Here's how the part is built. I have some questions about the finished solid (model axes, mm). A direction names the side the tool comes from. Coordinates: 2 decimals unless noted, no trailing zeros. Loops run counter-clockwise (first coordinate to the right, second up) from the corner with the lowest first, then second, coordinate; pieces in that order, holes last. Notation, with made-up numbers: (52, 67.5) -> (88, 67.5) arc R12 cw to (88, 88.5) -> close; hole circle Ø3 at (5, 21). An arc over 180 degrees is marked (long way). Answer as a JSON object with one key per item and string values. Group by question number.
Q1. I want a section at D-D on x = -6.5. Write out the boundary of the cut face in (y, z) (1 decimal), then the cut area to 3 significant figures.
Q2. On a 3-axis mill with a long thin cutter (end or side, diameter ignored), from which of +Z, -Z, +X, -X, +Y, -Y can I reach the whole of each face in a straight line? I mean faces 1 (the cylindrical face through (-2.75, 12.4, 21.57)), 2 (the cylindrical face through (-7.559, -5.796, 23.982)), 3 (the cylindrical face through (-0.69, 3.1, 9.08)). Say none if no direction works.
Q3. I'm going to push flat-ended pins straight in: pin 1 (5 mm diameter, centred on x = 3, z = 15.5, fed in from +Y); pin 2 (5 mm diameter, centred on y = -1.5, z = 6.5, fed in from -X) (3 decimals); pin 3 (8 mm diameter, centred on y = 7.5, z = 20, fed in from -X). Where does each tip first touch, or does it pass through?
Q4. I want a section at A-A on x = 0. Write out the boundary of the cut face in (y, z) (1 decimal).
Q5. I need wall thicknesses on line 1 (Z direction, x = -2.5, y = 2.75) (3 decimals); line 2 (Z direction, x = -2, y = -10); line 3 (Y direction, x = -1, z = 7.75). Which ranges of each line are inside material? Lowest first, please.
Q6. I want a section at C-C on z = 13.5. Write out the boundary of the cut face in (x, y) (3 decimals).
Autodesk Inventor part; units mm, degrees
ref_plane "YZ Plane" through (0, 0, 0) normal (1, 0, 0) x (0, 1, 0)
ref_plane "XZ Plane" through (0, 0, 0) normal (0, 1, 0) x (-1, 0, 0)
ref_plane "XY Plane" through (0, 0, 0) normal (0, 0, 1) x (1, 0, 0)
sketch "Sketch1" plane through (0, 0, 0) normal (0, 0, 1) x (1, 0, 0)
  circle A0 centre (0, 0) radius 3.175
  dimension "d0" = 6.35
extrude "Extrusion1" add sketch "Sketch1" along normal blind 18.415
sketch "Sketch2" plane through (0, 0, 18.415) normal (0, 0, 1) x (1, 0, 0)
  circle A0 centre (0, 0) radius 12.7
  dimension "d3" = 25.4
extrude "Extrusion2" add sketch "Sketch2" along normal blind 6.35
sketch "Sketch3" plane through (0, 0, 24.765) normal (0, 0, 1) x (1, 0, 0)
  circle A0 centre (0, 0) radius 9.525
  circle A1 centre (0, 0) radius 12.7
  dimension "d6" = 3.175
extrude "Extrusion3" cut sketch "Sketch3" against normal blind 1.5875
sketch "Sketch4" plane through (0, 0, 18.415) normal (0, 0, -1) x (-1, 0, 0)
  circle A0 centre (0, 0) radius 9.525
  circle A1 centre (0, 0) radius 12.7
  circle A2 centre (0, 0) radius 3.175
extrude "Extrusion4" cut sketch "Sketch4" against normal blind 1.5875 contours A1
properties part number "ScissorLiftSliderWheel"
Result set:
{
 "1": {"outline": "(-10.9, 20) -> (-7, 20) -> (-7, 18.4) -> (7, 18.4) -> (7, 20) -> (10.9, 20) -> (10.9, 23.2) -> (7, 23.2) -> (7, 24.8) -> (-7, 24.8) -> (-7, 23.2) -> (-10.9, 23.2) -> close", "area": "113 mm²"},
 "2": {"face 1": "+Z, -Z", "face 2": "+Z", "face 3": "-Z"},
 "3": {"pin 1": "stops at y = 3.14", "pin 2": "stops at x = -3.175", "pin 3": "stops at x = -12.21"},
 "4": {"outline": "(-12.7, 20) -> (-9.5, 20) -> (-9.5, 18.4) -> (-3.2, 18.4) -> (-3.2, 0) -> (3.2, 0) -> (3.2, 18.4) -> (9.5, 18.4) -> (9.5, 20) -> (12.7, 20) -> (12.7, 23.2) -> (9.5, 23.2) -> (9.5, 24.8) -> (-9.5, 24.8) -> (-9.5, 23.2) -> (-12.7, 23.2) -> close"},
 "5": {"line 1": "z = 18.415 to 24.765", "line 2": "z = 20 to 23.18", "line 3": "y = -3.01 to 3.01"},
 "6": {"outline": "circle Ø6.35 at (0, 0)"}
}
